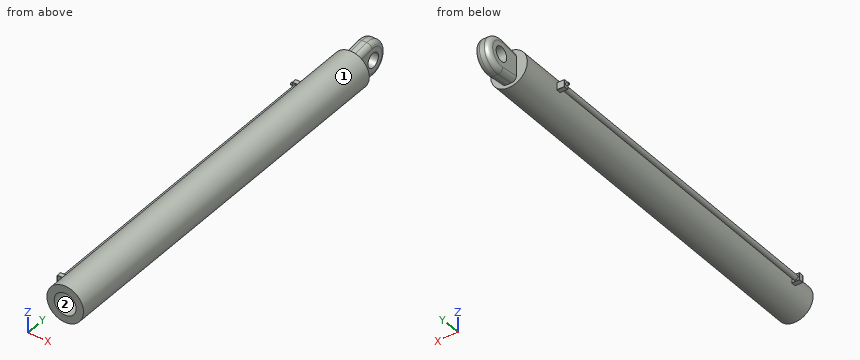
from build123d import *

# Parameters (mm, degrees)
SKETCH_1_R          = 75
SKETCH_1_R_2        = 45
EXTRUDE_1_DEPTH     = 1620
SKETCH_2_R          = 75
EXTRUDE_2_DEPTH     = 10
SKETCH_3_W          = 60
SKETCH_3_H          = 150
EXTRUDE_3_DEPTH     = 200
SKETCH_4_R          = 30
CUT_EXTRUDE_1_DEPTH = 1835.543539958
FILLET_1_R          = 20
EXTRUDE_4_DEPTH     = 20
SKETCH_6_R          = 10
EXTRUDE_5_DEPTH     = 660
SKETCH_10_R         = 5
SKETCH_10_R_2       = 2.5
EXTRUDE_6_DEPTH     = 10
FILLET_2_R          = 1


with BuildPart() as part:
    # 草图1 → 凸台-拉伸1 (new body)
    with BuildSketch(Plane(origin=(0, 0, 0), x_dir=(1, 0, 0), z_dir=(0, 1, 0))):
        with Locations(Location((0, 0, 0), (0, 0, 270))):
            Circle(SKETCH_1_R)
        with Locations(Location((0, 0, 0), (0, 0, 270))):
            Circle(SKETCH_1_R_2, mode=Mode.SUBTRACT)
    extrude(amount=EXTRUDE_1_DEPTH)

    # 草图2 → 凸台-拉伸2 (add)
    with BuildSketch(Plane(origin=(0, 1620, 0), x_dir=(1, 0, 0), z_dir=(0, 1, 0))):
        with Locations(Location((0, 0, 0), (0, 0, 270))):
            Circle(SKETCH_2_R)
    extrude(amount=EXTRUDE_2_DEPTH)

    # 草图3 → 凸台-拉伸3 (add)
    with BuildSketch(Plane(origin=(0, 1630, 0), x_dir=(1, 0, 0), z_dir=(0, 1, 0))):
        Rectangle(SKETCH_3_W, SKETCH_3_H)
    extrude(amount=EXTRUDE_3_DEPTH)

    # 草图4 → 切除-拉伸1 (cut, through all)
    with BuildSketch(Plane(origin=(30, 0, 0), x_dir=(0, 0, -1), z_dir=(1, 0, 0))):
        with Locations((0, 1715)):
            Circle(SKETCH_4_R)
        with BuildLine():
            Line((75, 1830), (75, 1630))
            Line((75, 1630), (60, 1630))
            Line((60, 1630), (69.468399859, 1706.389458724))
            ThreePointArc((69.468399859, 1706.389458724), (0, 1785), (-69.468399859, 1706.389458724))
            Line((-69.468399859, 1706.389458724), (-60, 1630))
            Line((-60, 1630), (-75, 1630))
            Line((-75, 1630), (-75, 1830))
            Line((-75, 1830), (75, 1830))
        make_face()
    extrude(amount=-CUT_EXTRUDE_1_DEPTH, mode=Mode.SUBTRACT)

    # 圆角1
    fillet_1_edges = [part.edges().sort_by_distance(p)[0] for p in [
        (-30, 1785, 0),
        (-30, 1668.194729362, 64.734199929),
        (-30, 1668.194729362, -64.734199929),
        (30, 1785, 0),
        (30, 1668.194729362, -64.734199929),
        (30, 1668.194729362, 64.734199929),
    ]]
    fillet(fillet_1_edges, radius=FILLET_1_R)

    # 草图5 → 凸台-拉伸4 (add)
    with BuildSketch(Plane(origin=(0, 100, 0), x_dir=(-1, 0, 0), z_dir=(0, -1, 0))):
        with BuildLine():
            Line((73.484692283, 15), (105, 15))
            Line((105, 15), (105, -15))
            Line((105, -15), (73.484692283, -15))
            ThreePointArc((73.484692283, -15), (75, 0), (73.484692283, 15))
        make_face()
    extrude_4 = extrude(amount=-EXTRUDE_4_DEPTH)

    # 草图6 → 凸台-拉伸5 (add)
    with BuildSketch(Plane(origin=(0, 120, 0), x_dir=(-1, 0, 0), z_dir=(0, -1, 0))):
        with Locations(Location((89.242346142, 0, 0), (0, 0, 90))):
            Circle(SKETCH_6_R)
    extrude_5 = extrude(amount=-EXTRUDE_5_DEPTH)

    # 镜向2: 凸台-拉伸4, 凸台-拉伸5 across plane
    add(extrude_4.mirror(Plane(origin=(-89.242346142, 780, 0), x_dir=(0, 0, 1), z_dir=(0, -1, 0))))
    add(extrude_5.mirror(Plane(origin=(-89.242346142, 780, 0), x_dir=(0, 0, 1), z_dir=(0, -1, 0))))

    # 草图10 → 凸台-拉伸6 (add)
    with BuildSketch(Plane.ZY.offset(105)):
        with Locations(Location((0, 1450, 0), (0, 0, 180))):
            Circle(SKETCH_10_R)
        with Locations((0, 1450)):
            Circle(SKETCH_10_R_2, mode=Mode.SUBTRACT)
    extrude(amount=EXTRUDE_6_DEPTH)

    # 圆角2
    fillet_2_edges = [part.edges().sort_by_distance(p)[0] for p in [
        (-89.242346142, 1440, 15),
        (-105, 1450, 15),
        (-89.242346142, 1460, 15),
        (-105, 1440, 0),
        (-89.242346142, 1440, -15),
        (-105, 1450, -15),
        (-105, 1460, 0),
        (-89.242346142, 1460, -15),
        (-89.242346142, 100, 15),
        (-89.242346142, 120, 15),
        (-105, 100, 0),
        (-89.242346142, 100, -15),
        (-89.242346142, 120, -15),
        (-105, 120, 0),
        (-105, 110, -15),
    ]]
    fillet(fillet_2_edges, radius=FILLET_2_R)


solid = part.part
Could you check a few things on this model? Use its own coordinates, in mm. Face numbers are marked on the shaded views. Give positions to 0.01 mm unless a question says otherwise; leave off trailing zeros. Write each loop counter-clockwise with the first axis right and the second up, starting at its lowest first coordinate (ties: lowest second). Pieces come first, ordered by that corner, then holes. Notation, with made-up numbers: (78, 7) -> (94, 7) arc R13 ccw to (94, 12) -> close; hole circle Ø4 at (83, 18). An arc over 180 degrees is marked (long way). Write each question's results on one line, items separated by ' | '. Start each with the question number.
Q1. Suppose I cut it at B-B, the plane y = 1074.5. List the corners of the cut face in (x, z) for me.
Q2. I need wall thicknesses on probe 1 along X at (y, z) = (891, 0); probe 2 along Z at (x, y) = (-107, 1450); probe 3 along Z at (x, y) = (2.5, 250.5). Which ranges of each line are inside material? Lowest first, please.
Q3. We'd pull the mould along Z, two halves only. Please class the marked faces 1 and 2: +Z half, -Z half, draft (parallel to the pull), parting line (faces both ways), or undercut.
Q4. Suppose I cut it at A-A, the plane y = 1477. List the corners of the cut face in (x, z) for me, and give its area (3 significant figures).
Q5. I'm going to push flat-ended pins straight in: pin 1 Ø1 at (y, z) = (447, -49) entering from -X; pin 2 Ø20 at (x, y) = (-87.5, 1445.5) entering from -Z; pin 3 Ø1 at (x, y) = (-44, 474) entering from +Z. Where does each tip first touch, or does it pass through?
Outcome:
1) outline: circle Ø20 at (-89.24, 0); circle Ø150 at (0, 0); hole circle Ø90 at (0, 0)
2) probe 1: -99.24 to -79.24, -75 to -45, 45 to 75 | probe 2: -5 to -2.5, 2.5 to 5 | probe 3: -74.96 to -44.93, 44.93 to 74.96
3) face 1: parting line | face 2: undercut
4) outline: circle Ø150 at (0, 0); hole circle Ø90 at (0, 0) | area: 11,300 mm2
5) pin 1: x = -57.21 | pin 2: z = -15 | pin 3: z = 61.1
